For this review, take the finished solid that the model builds, in its own axes (mm). Face numbers are marked on the shaded views. A direction names the side the tool comes from. Give positions to 0.01 mm unless a question says otherwise; leave off trailing zeros. Write each loop counter-clockwise with the first axis right and the second up, starting at its lowest first coordinate (ties: lowest second). Pieces come first, ordered by that corner, then holes. Notation, with made-up numbers: M 66,36.25 L 106,36.25 A37 ccw 106,75.25 Z; hole C 32,53.5 d9. An arc over 180 degrees is marked long. Write item = value, one per line.
```python
from build123d import *

# Parameters (mm, degrees)
BOSS_EXTRUDE1_DEPTH                      = 63.5
F_5_16_0_3125_DIAMETER_HOLE1_D           = 7.9375
F_5_16_0_3125_DIAMETER_HOLE1_ON_FACE_2_D = 7.9375


with BuildPart() as part:
    # Sketch3 → Boss-Extrude1 (new body)
    with BuildSketch(Plane.XY):
        with BuildLine():
            Line((0, 6.35), (0, 33.655))
            ThreePointArc((0, 33.655), (-0.371974388, 34.553025612), (-1.27, 34.925))
            Line((-1.27, 34.925), (-3.175, 34.925))
            Line((-3.175, 34.925), (-3.175, 0))
            ThreePointArc((-3.175, 0), (-2.24506403, -2.24506403), (0, -3.175))
            Line((0, -3.175), (34.925, -3.175))
            Line((34.925, -3.175), (34.925, -1.27))
            ThreePointArc((34.925, -1.27), (34.553025612, -0.371974388), (33.655, 0))
            Line((33.655, 0), (6.35, 0))
            ThreePointArc((6.35, 0), (1.859871939, 1.859871939), (0, 6.35))
        make_face()
    extrude(amount=BOSS_EXTRUDE1_DEPTH)

    # 5/16 (0.3125) Diameter Hole1 (through all)
    with Locations(Plane(origin=(22.225, 0, 53.975), x_dir=(1, 0, 0), z_dir=(0, 1, 0))):
        with Locations((0, 0), (0, 44.45)):
            Hole(F_5_16_0_3125_DIAMETER_HOLE1_D / 2)

    # 5/16 (0.3125) Diameter Hole1 on face 2 (through all)
    with Locations(Plane(origin=(0, 22.225, 9.525), x_dir=(0, 0, 1), z_dir=(1, 0, 0))):
        with Locations((0, 0), (44.45, 0)):
            Hole(F_5_16_0_3125_DIAMETER_HOLE1_ON_FACE_2_D / 2)


solid = part.part
```
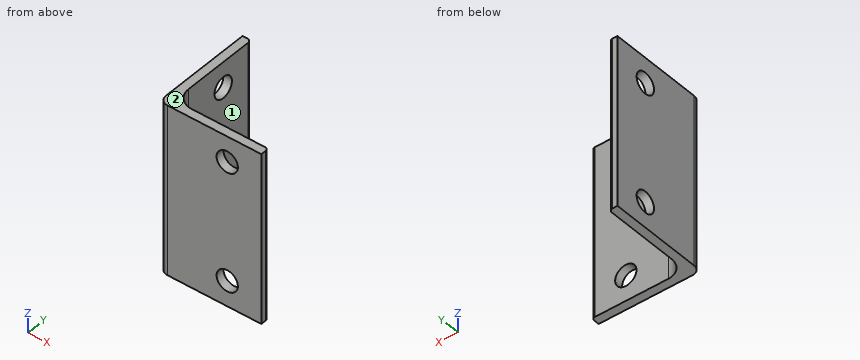
1. We need section A-A, the plane z = 27.5. Write out the cut boundary in (x, y) (3 decimals), then the cut area to 3 significant figures.
Responses:
outline = M -3.175,0 A3.175 ccw 0,-3.175 L 34.925,-3.175 L 34.925,-1.27 A1.27 ccw 33.655,0 L 6.35,0 A6.35 cw 0,6.35 L 0,33.655 A1.27 ccw -1.27,34.925 L -3.175,34.925 Z
area = 238 mm2
2. We need section C-C, the plane y = 23. Write out the cut boundary in (x, z) (3 decimals).
Responses:
outline = M -3.175,0 L 0,0 L 0,5.633 L -3.175,5.633 Z; M -3.175,13.417 L 0,13.417 L 0,50.083 L -3.175,50.083 Z; M -3.175,57.867 L 0,57.867 L 0,63.5 L -3.175,63.5 Z
3. We need section D-D, the plane y = 30.5. Write out the cut boundary in (x, z) (3 decimals).
Responses:
outline = M -3.175,0 L 0,0 L 0,63.5 L -3.175,63.5 Z
4. Insertion check: P1, Ø6.5, axis at y = 22.225, z = 9.525, coming from the +X side; P2, Ø1.5, axis at y = 8, z = 55.5, coming from the +X side; P3, Ø12, axis at x = 8, z = 44.5, coming from the +Y side; P4, Ø5, axis at x = 9, y = 2, coming from the +Z side. Each pin has a flat end and moves straight along its axis. Give the tip position at first contact, or say it passes through.
Responses:
P1 = through
P2 = 0
P3 = 1.72
P4 = 63.5
5. We need section B-B, the plane x = 19. Write out the cut boundary in (y, z) (3 decimals).
Responses:
outline = M -3.175,0 L 0,0 L 0,7.212 L -3.175,7.212 Z; M -3.175,11.838 L 0,11.838 L 0,51.662 L -3.175,51.662 Z; M -3.175,56.288 L 0,56.288 L 0,63.5 L -3.175,63.5 Z
6. Machinability: for the marked faces 1 and 2, which of the approach directions +Z, -Z, +X, -X, +Y, -Y give a long, thin tool a straight path to every point of the face, cutting with its end or side? Answer none if there is none.
Responses:
face_1 = +Z, -Z, +X, +Y
face_2 = +Z, +X, -X, +Y, -Y
7. For line 1 along X through (y, z) = (26.5, 53) (3 decimals); line 2 along X through (y, z) = (2, 10.5) (3 decimals), list the stretches that pass through material, from the lowest coordinate up. Write a range as from..to.
Responses:
line_1 = -3.175..0
line_2 = -3.175..1.724
